Work out the finished part from the listing and answer in its coordinate system (mm). A direction names the side the tool comes from. Give positions to 0.01 mm unless a question says otherwise; leave off trailing zeros. Loops run counter-clockwise (first coordinate to the right, second up) from the corner with the lowest first, then second, coordinate; pieces in that order, holes last. Notation, with made-up numbers: (4, 17) -> (24, 17) arc R24 ccw to (24, 48) -> close; hole circle Ø4 at (30, 3). An arc over 180 degrees is marked (long way). Answer as CSV lines item,"result". Start each with the question number.
1. Determine the mould class of faces 3 (the face through (-11.077, -68.196, 1.673)), 4 (the face through (-11.077, -1.804, 1.673)), 5 (the face through (-3.679, -55.026, 9.857)), 6 (the face through (-3, -35, 3.3)) for opening direction Y: +Y half, -Y half, draft (parallel to the pull), parting line (faces both ways), or undercut.
2. A tool of negligible diameter and unlimited length cuts with its end or side. For faces 1 (the face through (-3, -12, 16.6)), 2 (the face through (-0.427, -11.099, 9.857)), from which of +Z, -Z, +X, -X, +Y, -Y can it reach the whole face along a straight path? Write none if from no direction.
3. Find section D-D, the plane y = -13. Give the vertices of the cut face in (x, z).
4. Find section B-B, the plane z = 14. Give the vertices of the cut face in (x, y).
5. Find the intervals of material crossed by line 1 along Y through (x, z) = (-3.5, 11); line 2 along Z through (x, y) = (0, -22.5); line 3 along X through (y, z) = (-56, 7), in increasing order.
6. Find section C-C, the plane x = -1. Give the vertices of the cut face in (y, z).
7. Find section A-A, the plane y = -58. Give the vertices of the cut face in (x, z).
8. Flat-ended cylindrical pins translate along their axes: pin 1 Ø2 at (x, y) = (-5, -27) entering from -Z; pin 2 Ø5 at (x, z) = (-7, 8) entering from +Y; pin 3 Ø1.5 at (x, z) = (-0.5, 13) entering from -Y; pin 4 Ø1.5 at (x, y) = (-0.5, -61.5) entering from +Z. Find the tip coordinate at first contact, or state that the pin passes through.
from build123d import *

# Parameters (mm, degrees)
F0_W     = 20
F0_H     = 3.3
F1_DEPTH = 70
F2_R     = 3
F3_DEPTH = 13.3
F4_R     = 6


with BuildPart() as f1:
    # F0 (on Front) → F1 (new body)
    with BuildSketch(Plane.XZ):
        with Locations((-2.78839, 1.65)):
            Rectangle(F0_W, F0_H)
    extrude(amount=F1_DEPTH)

    # F2 (on face) → F3 (join)
    with BuildSketch(Plane.XY.offset(3.3)):
        with Locations((-3.28839, -12)):
            Circle(F2_R)
        with Locations((-3.28839, -58)):
            Circle(F2_R)
    extrude(amount=F3_DEPTH)

    # F4
    f4_edges = [f1.edges().sort_by_distance(p)[0] for p in [
        (-12.78839, 0, 1.65),
        (-12.78839, -70, 1.65),
    ]]
    fillet(f4_edges, radius=F4_R)


solid = f1.part
Resolved:
1,face 3,"-Y half"
1,face 4,"+Y half"
1,face 5,"undercut"
1,face 6,"undercut"
2,face 1,"+Z, +X, -X, +Y, -Y"
2,face 2,"+Z"
3,outline,"(-12.79, 0) -> (7.21, 0) -> (7.21, 3.3) -> (-0.46, 3.3) -> (-0.46, 16.6) -> (-6.12, 16.6) -> (-6.12, 3.3) -> (-12.79, 3.3) -> close"
4,outline,"circle Ø6 at (-3.29, -58); circle Ø6 at (-3.29, -12)"
5,line 1,"y = -60.99 to -55.01, -14.99 to -9.01"
5,line 2,"z = 0 to 3.3"
5,line 3,"x = -5.52 to -1.05"
6,outline,"(-70, 0) -> (0, 0) -> (0, 3.3) -> (-10.06, 3.3) -> (-10.06, 16.6) -> (-13.94, 16.6) -> (-13.94, 3.3) -> (-56.06, 3.3) -> (-56.06, 16.6) -> (-59.94, 16.6) -> (-59.94, 3.3) -> (-70, 3.3) -> close"
7,outline,"(-12.79, 0) -> (7.21, 0) -> (7.21, 3.3) -> (-0.29, 3.3) -> (-0.29, 16.6) -> (-6.29, 16.6) -> (-6.29, 3.3) -> (-12.79, 3.3) -> close"
8,pin 1,"stops at z = 0"
8,pin 2,"stops at y = -9.26"
8,pin 3,"stops at y = -60.2"
8,pin 4,"stops at z = 3.3"
